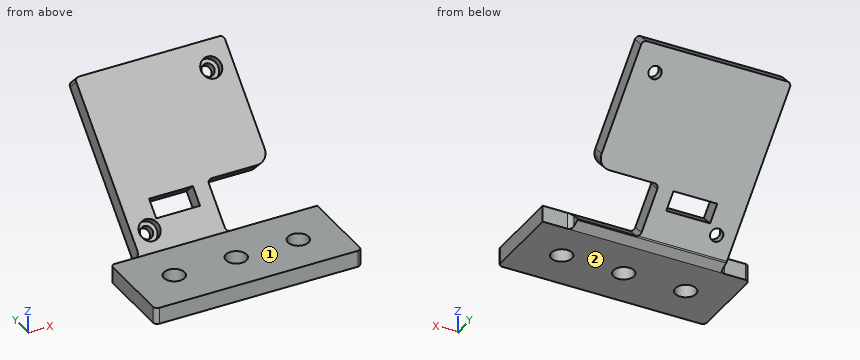
```python
from build123d import *

# Parameters (mm, degrees)
SKETCH_1_W          = 50
SKETCH_1_H          = 20
EXTRUDE_1_DEPTH     = 4
EXTRUDE_2_DEPTH     = 18
SKETCH_5_R          = 1.5
CUT_EXTRUDE_1_DEPTH = 59.543629581
SKETCH_6_W          = 15
SKETCH_6_H          = 12
CUT_EXTRUDE_2_DEPTH = 59.543629581
FILLET_1_R          = 1
FILLET_2_R          = 1
FILLET_3_R          = 1
SKETCH_7_R          = 2.5
CUT_EXTRUDE_3_DEPTH = 2
SKETCH_8_R          = 2.5
CUT_EXTRUDE_4_DEPTH = 57.695644481
SKETCH_9_W          = 10.6
SKETCH_9_H          = 4.503957044
CUT_EXTRUDE_5_DEPTH = 10
FILLET_4_R          = 3


with BuildPart() as part:
    # 草图1 → 凸台-拉伸1 (new body)
    with BuildSketch(Plane.XY):
        Rectangle(SKETCH_1_W, SKETCH_1_H)
    extrude(amount=EXTRUDE_1_DEPTH)

    # 草图4 → 凸台-拉伸2 (add, symmetric)
    with BuildSketch(Plane(origin=(0, 0, 0), x_dir=(0, 0, -1), z_dir=(1, 0, 0))):
        Polygon((-4, 10), (-32.991378029, 38.991378029), (-30.162950904, 41.819805153), (-1.087902103, 12.744756352), (0, 10), align=None)
    extrude(amount=EXTRUDE_2_DEPTH, both=True)

    # 草图5 → 切除-拉伸1 (cut, through all)
    with BuildSketch(Plane(origin=(0, 3, -3), x_dir=(1, 0, 0), z_dir=(0, -0.7071067811865488, 0.7071067811865462))):
        with Locations(Location((12.721590614, 44.887973136, 0), (0, 0, 270))):
            Circle(SKETCH_5_R)
        with Locations(Location((-13.670456314, 14.830364134, 0), (0, 0, 270))):
            Circle(SKETCH_5_R)
    extrude(amount=-CUT_EXTRUDE_1_DEPTH, mode=Mode.SUBTRACT)

    # 草图6 → 切除-拉伸2 (cut, through all)
    with BuildSketch(Plane(origin=(0, 3, -3), x_dir=(1, 0, 0), z_dir=(0, -0.7071067811865488, 0.7071067811865462))):
        with Locations((10.5, 15.899494937)):
            Rectangle(SKETCH_6_W, SKETCH_6_H)
    extrude(amount=-CUT_EXTRUDE_2_DEPTH, mode=Mode.SUBTRACT)

    # 圆角1
    fillet_1_edges = [part.edges().sort_by_distance(p)[0] for p in [
        (3, 11.414213562, 2.585786438),
        (3, 19.899494937, 11.071067812),
    ]]
    fillet(fillet_1_edges, radius=FILLET_1_R)

    # 圆角2
    # the kernel refuses this fillet: 1 mm, written as the material it adds along each edge
    with BuildSketch(Plane(origin=(-18, 10, 0), x_dir=(0, 1, 0), z_dir=(0, 0, 1))) as fillet_2_piece_1_section:
        with BuildLine():
            CenterArc((FILLET_2_R, FILLET_2_R), FILLET_2_R, 180, 90)
            Line((0, FILLET_2_R), (0, 0))
            Line((0, 0), (FILLET_2_R, 0))
        make_face()
    fillet_2_piece_1 = extrude(amount=4, mode=Mode.PRIVATE)
    fillet_2_piece_1 = split(fillet_2_piece_1, bisect_by=Plane(origin=(-18.229103678, 9.132725648, 3.132725648), z_dir=(0, 0.7071067811865489, -0.7071067811865462)), keep=Keep.TOP, mode=Mode.PRIVATE)
    fillet_2_piece_1 = split(fillet_2_piece_1, bisect_by=Plane(origin=(-18.229103678, 10.891700331, 0.353431249), z_dir=(0, -0.36846891223412287, 0.9296400705203075)), keep=Keep.TOP, mode=Mode.PRIVATE)
    add(fillet_2_piece_1)
    with BuildSketch(Plane(origin=(-18, 10, 0), x_dir=(0, 1, 0), z_dir=(0, 0, 1))) as fillet_2_piece_2_section:
        with BuildLine():
            CenterArc((FILLET_2_R, FILLET_2_R), FILLET_2_R, 180, 90)
            Line((0, FILLET_2_R), (0, 0))
            Line((0, 0), (FILLET_2_R, 0))
        make_face()
    fillet_2_piece_2 = extrude(amount=6.5, mode=Mode.PRIVATE)
    fillet_2_piece_2 = split(fillet_2_piece_2, bisect_by=Plane(origin=(-18.106472513, 10.430118052, 4), z_dir=(0, 0, 1)), keep=Keep.TOP, mode=Mode.PRIVATE)
    fillet_2_piece_2 = split(fillet_2_piece_2, bisect_by=Plane(origin=(-18.106472513, 10.322588538, 4.322588538), z_dir=(0, 0.7071067811865489, -0.7071067811865462)), keep=Keep.TOP, mode=Mode.PRIVATE)
    add(fillet_2_piece_2)
    with BuildSketch(Plane(origin=(18, 10, 0), x_dir=(0, 1, 0), z_dir=(0, 0, 1))) as fillet_2_piece_3_section:
        with BuildLine():
            CenterArc((FILLET_2_R, -FILLET_2_R), FILLET_2_R, 90, 90)
            Line((0, -FILLET_2_R), (0, 0))
            Line((0, 0), (FILLET_2_R, 0))
        make_face()
    fillet_2_piece_3 = extrude(amount=4, mode=Mode.PRIVATE)
    fillet_2_piece_3 = split(fillet_2_piece_3, bisect_by=Plane(origin=(18.236725667, 10.843896017, 0.334483697), z_dir=(0, -0.36846891223412287, 0.9296400705203075)), keep=Keep.TOP, mode=Mode.PRIVATE)
    fillet_2_piece_3 = split(fillet_2_piece_3, bisect_by=Plane(origin=(18.236725667, 11.136071068, 2.863928932), z_dir=(0, -0.7071067811865462, -0.7071067811865489)), keep=Keep.TOP, mode=Mode.PRIVATE)
    add(fillet_2_piece_3)
    # the kernel refuses this fillet: 1 mm, written as the material it takes off along each edge
    with BuildSketch(Plane(origin=(-18, 37.223611076, 34.759144982), x_dir=(1, 0, 0), z_dir=(0, 0.7071067811865485, -0.7071067811865467)), Plane(origin=(18, 37.223611076, 34.759144982), x_dir=(0, -0.7071067811865467, -0.7071067811865485), z_dir=(0, 0.7071067811865485, -0.7071067811865467))) as fillet_2_2_piece_1:
        with BuildLine():
            CenterArc((FILLET_2_R, FILLET_2_R), FILLET_2_R, 180, 90)
            Line((0, FILLET_2_R), (0, 0))
            Line((0, 0), (FILLET_2_R, 0))
        make_face()
    extrude(amount=9, mode=Mode.SUBTRACT)
    with BuildSketch(Plane(origin=(-25, 10, -2.5), x_dir=(1, 0, 0), z_dir=(0, 0, 1)), Plane(origin=(25, -10, -2.5), x_dir=(-1, 0, 0), z_dir=(0, 0, 1)), Plane(origin=(-25, -10, -2.5), x_dir=(0, 1, 0), z_dir=(0, 0, 1))) as fillet_2_2_piece_2:
        with BuildLine():
            CenterArc((FILLET_2_R, -FILLET_2_R), FILLET_2_R, 90, 90)
            Line((0, -FILLET_2_R), (0, 0))
            Line((0, 0), (FILLET_2_R, 0))
        make_face()
    extrude(amount=9, mode=Mode.SUBTRACT)

    # 圆角3
    fillet_3_edges = [part.edges().sort_by_distance(p)[0] for p in [
        (0, 12.744756352, 1.087902103),
    ]]
    fillet(fillet_3_edges, radius=FILLET_3_R)

    # 草图7 → 切除-拉伸3 (cut)
    with BuildSketch(Plane(origin=(0, 3, -3), x_dir=(1, 0, 0), z_dir=(0, -0.7071067811865488, 0.7071067811865462))):
        with Locations(Location((12.721590614, 44.887973136, 0), (0, 0, 270))):
            Circle(SKETCH_7_R)
        with Locations(Location((-13.670456314, 14.830364134, 0), (0, 0, 270))):
            Circle(SKETCH_7_R)
    extrude(amount=-CUT_EXTRUDE_3_DEPTH, mode=Mode.SUBTRACT)

    # 草图8 → 切除-拉伸4 (cut, through all)
    with BuildSketch(Plane.XY.offset(4)):
        Circle(SKETCH_8_R)
        with Locations((15, 0)):
            Circle(SKETCH_8_R)
        with Locations((-15, 0)):
            Circle(SKETCH_8_R)
    extrude(amount=-CUT_EXTRUDE_4_DEPTH, mode=Mode.SUBTRACT)

    # 草图9 → 切除-拉伸5 (cut)
    with BuildSketch(Plane(origin=(0, 3, -3), x_dir=(1, 0, 0), z_dir=(0, -0.7071067811865488, 0.7071067811865462))):
        with Locations((-6, 19.119035577)):
            Rectangle(SKETCH_9_W, SKETCH_9_H)
    extrude(amount=-CUT_EXTRUDE_5_DEPTH, mode=Mode.SUBTRACT)

    # 圆角4
    fillet_4_edges = [part.edges().sort_by_distance(p)[0] for p in [
        (18, 19.899494937, 11.071067812),
    ]]
    fillet(fillet_4_edges, radius=FILLET_4_R)


solid = part.part
```
The listing builds one solid part. Answer for the finished solid, in the listing's coordinates (mm). Face numbers are marked on the shaded views. A direction names the side the tool comes from. Give positions to 0.01 mm unless a question says otherwise; leave off trailing zeros. Order: outer loops, then holes, each group sorted by start corner. A loop starts at its lowest first (then second) coordinate and runs counter-clockwise, first axis right, second up.
1) Given P1, Ø3, axis at x = -22, z = 1, coming from the +Y side; P2, Ø1.8, axis at y = 16.5, z = 9.5, coming from the -X side; P3, Ø10, axis at x = 14.5, z = 14, coming from the +Y side, each flat-ended and moving along its own axis, determine where each tip first touches the part or whether it passes through.
Reported:
P1: stops at y = 10
P2: stops at x = -18
P3: stops at y = 30.66
2) Consider line 1 along Y through (x, z) = (15, 1.9); line 2 along Z through (x, y) = (-20, 3); line 3 along X through (y, z) = (14.5, 4). Determine where each line is inside the solid, lowest interval first.
Reported:
line 1: y = -10 to -2.5, 2.5 to 12.1
line 2: z = 0 to 4
line 3: x = -18 to 3
3) Find section B-B on y = 0. Write down the section's boundary in (x, z), then the cut area to 3 significant figures.
Reported:
outline: (-25, 0) - (-17.5, 0) - (-17.5, 4) - (-25, 4) - close; (-12.5, 0) - (-2.5, 0) - (-2.5, 4) - (-12.5, 4) - close; (2.5, 0) - (12.5, 0) - (12.5, 4) - (2.5, 4) - close; (17.5, 0) - (25, 0) - (25, 4) - (17.5, 4) - close
area: 140 mm2
4) Find section A-A on x = 0. Write down the section's boundary in (y, z), then the cut area to 3 significant figures.
Reported:
outline: (-10, 0) - (-2.5, 0) - (-2.5, 4) - (-10, 4) - close; (2.5, 0) - (10, 0) - (12.55, 1.01) arc R1 ccw to (12.89, 1.23) - (41.82, 30.16) - (38.99, 32.99) - (10, 4) - (2.5, 4) - close
area: 230 mm2
5) For the marked faces 1 and 2, determine the directions among +Z, -Z, +X, -X, +Y, -Y from which every point of the face is accessible in a straight line to the end or side of a thin tool.
Reported:
face 1: +Z, +X, -X, -Y
face 2: -Z, +X, -X, +Y, -Y
6) Find section D-D on x = -6. Write down the section's boundary in (y, z), then the cut area to 3 significant figures.
Reported:
outline: (-10, 0) - (10, 0) - (12.55, 1.01) arc R1 ccw to (12.89, 1.23) - (17.76, 6.1) - (14.93, 8.93) - (10, 4) - (-10, 4) - close; (18.11, 12.11) - (20.94, 9.28) - (41.82, 30.16) - (38.99, 32.99) - close
area: 232 mm2
7) Find section C-C on x = -14.5. Write down the section's boundary in (y, z), then the cut area to 3 significant figures.
Reported:
outline: (-10, 0) - (-2.45, 0) - (-2.45, 4) - (-10, 4) - close; (2.45, 0) - (10, 0) - (12.55, 1.01) arc R1 ccw to (12.89, 1.23) - (15.43, 3.77) - (14.02, 5.19) - (13.23, 4.4) - (11.82, 5.82) - (10, 4) - (2.45, 4) - close; (15.15, 9.15) - (16.57, 7.74) - (15.78, 6.96) - (17.2, 5.54) - (41.82, 30.16) - (38.99, 32.99) - close
area: 216 mm2
